The model under review builds one solid part; all positions refer to its coordinate system, in mm. A direction names the side the tool comes from. Give positions to 0.01 mm unless a question says otherwise; leave off trailing zeros. Loops run counter-clockwise (first coordinate to the right, second up) from the corner with the lowest first, then second, coordinate; pieces in that order, holes last. Notation, with made-up numbers: M 3,28.5 L 54,28.5 A25 ccw 54,49.5 Z; hole C -36,77 d6. An arc over 180 degrees is marked long. Put each result on its own line as item: value. Start each with the question number.
```python
from build123d import *

# Parameters (mm, degrees)
SKETCH1_R                     = 3.175
BOSS_EXTRUDE2_DEPTH           = 76.2
SKETCH1_5_R                   = 3.175
BOSS_EXTRUDE3_DEPTH           = 6.35
SKETCH5_R                     = 3.175
BOSS_EXTRUDE4_DEPTH           = 6.35
SKETCH6_W                     = 50.8
SKETCH6_H                     = 50.8
CUT_EXTRUDE1_DEPTH            = 21.59
SKETCH7_W                     = 5.86068256
SKETCH7_H                     = 10.16
BOSS_EXTRUDE5_DEPTH           = 21.59
BOSS_EXTRUDE5_DRAFT           = 5
BOSS_EXTRUDE5_PROFILE_2_DEPTH = 21.59
BOSS_EXTRUDE5_PROFILE_2_DRAFT = 5
BOSS_EXTRUDE5_PROFILE_3_DEPTH = 21.59
BOSS_EXTRUDE5_PROFILE_3_DRAFT = 5
BOSS_EXTRUDE5_PROFILE_4_DEPTH = 21.59
BOSS_EXTRUDE5_PROFILE_4_DRAFT = 5
BOSS_EXTRUDE5_PROFILE_5_DEPTH = 21.59
BOSS_EXTRUDE5_PROFILE_5_DRAFT = 5
SKETCH10_R                    = 36.051864109
CUT_EXTRUDE2_DEPTH            = 21.59


with BuildPart() as part:
    # Sketch1 → Boss-Extrude2 (new body)
    with BuildSketch(Plane(origin=(0, 0, 0), x_dir=(1, 0, 0), z_dir=(0, 1, 0))):
        with BuildLine():
            Line((-4.208751998, -43.475305064), (45.017746951, 2.631829887))
            Line((45.017746951, 2.631829887), (35.550660053, 36.209226482))
            ThreePointArc((35.550660053, 36.209226482), (39.762177432, 42.05307025), (33.11828595, 44.83625091))
            Line((33.11828595, 44.83625091), (15.243844224, 108.232438689))
            Line((15.243844224, 108.232438689), (-2.783728935, 127.479661752))
            Line((-2.783728935, 127.479661752), (3.678966496, 133.532831827))
            Line((3.678966496, 133.532831827), (-3.005742225, 140.669792455))
            Line((-3.005742225, 140.669792455), (-9.468437655, 134.61662238))
            Line((-9.468437655, 134.61662238), (-27.496010814, 153.863845442))
            Line((-27.496010814, 153.863845442), (-74.966911398, 109.401060841))
            Line((-74.966911398, 109.401060841), (-32.227053049, 63.769650553))
            Line((-32.227053049, 63.769650553), (-4.208751998, -43.475305064))
        make_face()
        with Locations(Location((35.334305242, 40.804639607, 0), (0, 0, 90))):
            Circle(SKETCH1_R, mode=Mode.SUBTRACT)
        with BuildLine():
            Line((-27.946524097, 65.532765046), (-68.844709626, 109.197904706))
            Line((-68.844709626, 109.197904706), (-27.496010814, 147.926436632))
            Line((-27.496010814, 147.926436632), (12.111157264, 105.390011693))
            Line((12.111157264, 105.390011693), (34.544848217, 24.491577435))
            ThreePointArc((34.544848217, 24.491577435), (36.285698832, 19.303992732), (36.875100326, 13.863937421))
            ThreePointArc((36.875100326, 13.863937421), (14.585843996, -11.34485616), (-13.162952731, 7.689284266))
            Line((-13.162952731, 7.689284266), (-27.946524097, 65.532765046))
        make_face(mode=Mode.SUBTRACT)
        with Locations(Location((-2.894634056, 134.074815557, 0), (0, 0, 90))):
            Circle(SKETCH1_R, mode=Mode.SUBTRACT)
    extrude(amount=BOSS_EXTRUDE2_DEPTH)

    # Sketch1_5 → Boss-Extrude3 (add)
    with BuildSketch(Plane(origin=(0, 0, 0), x_dir=(1, 0, 0), z_dir=(0, 1, 0))):
        with BuildLine():
            Line((-27.496010814, 147.926436632), (-68.844709626, 109.197904706))
            Line((-68.844709626, 109.197904706), (-27.946524097, 65.532765046))
            Line((-27.946524097, 65.532765046), (-13.162952731, 7.689284266))
            ThreePointArc((-13.162952731, 7.689284266), (3.03743719, 37.821521623), (34.544848217, 24.491577435))
            Line((34.544848217, 24.491577435), (12.111157264, 105.390011693))
            Line((12.111157264, 105.390011693), (-27.496010814, 147.926436632))
        make_face()
        with Locations(Location((-32.808552916, 77.429328599, 0), (0, 0, 270))):
            Circle(SKETCH1_5_R, mode=Mode.SUBTRACT)
        with Locations(Location((-1.199981142, 109.041759799, 0), (0, 0, 270))):
            Circle(SKETCH1_5_R, mode=Mode.SUBTRACT)
    extrude(amount=BOSS_EXTRUDE3_DEPTH)

    # Sketch5 → Boss-Extrude4 (add)
    with BuildSketch(Plane(origin=(0, 76.2, 0), x_dir=(1, 0, 0), z_dir=(0, 1, 0))):
        with BuildLine():
            Line((45.017746951, 2.631829887), (35.550660053, 36.209226482))
            ThreePointArc((35.550660053, 36.209226482), (39.762177432, 42.05307025), (33.11828595, 44.83625091))
            Line((33.11828595, 44.83625091), (15.243844224, 108.232438689))
            Line((15.243844224, 108.232438689), (-2.783728935, 127.479661752))
            Line((-2.783728935, 127.479661752), (3.678966496, 133.532831827))
            Line((3.678966496, 133.532831827), (-3.005742225, 140.669792455))
            Line((-3.005742225, 140.669792455), (-9.468437655, 134.61662238))
            Line((-9.468437655, 134.61662238), (-27.496010814, 153.863845442))
            Line((-27.496010814, 153.863845442), (-74.966911398, 109.401060841))
            Line((-74.966911398, 109.401060841), (-32.227053049, 63.769650553))
            Line((-32.227053049, 63.769650553), (-4.208751998, -43.475305064))
            Line((-4.208751998, -43.475305064), (45.017746951, 2.631829887))
        make_face()
        with Locations(Location((-2.894634056, 134.074815557, 0), (0, 0, 90))):
            Circle(SKETCH5_R, mode=Mode.SUBTRACT)
        with Locations(Location((35.334305242, 40.804639607, 0), (0, 0, 90))):
            Circle(SKETCH5_R, mode=Mode.SUBTRACT)
    extrude(amount=BOSS_EXTRUDE4_DEPTH)

    # Sketch6 → Cut-Extrude1 (cut)
    with BuildSketch(Plane(origin=(14.64974053, 0, -13.721421958), x_dir=(0.683604049055853, 0, 0.729853070223345), z_dir=(-0.729853070223345, 0, 0.683604049055853))):
        with Locations((-99.833701757, 41.275)):
            Rectangle(SKETCH6_W, SKETCH6_H)
    extrude(amount=-CUT_EXTRUDE1_DEPTH, mode=Mode.SUBTRACT)


with BuildPart() as boss_extrude5_tool:
    # Sketch7 → Boss-Extrude5 (with draft: the straight prism first)
    with BuildSketch(Plane(origin=(14.64974053, 0, -13.721421958), x_dir=(0.683604049055853, 0, 0.729853070223345), z_dir=(-0.729853070223345, 0, 0.683604049055853))):
        with Locations((-128.164043037, 77.47)):
            Rectangle(SKETCH7_W, SKETCH7_H)
    extrude(amount=BOSS_EXTRUDE5_DEPTH)
    # Boss-Extrude5: the draft: its side faces are tilted about the plane it starts from
    boss_extrude5_sides = [boss_extrude5_tool.faces().sort_by_distance(p)[0] for p in [
        (-82.845675291, 77.47, -102.021555132),
        (-80.842482126, 72.39, -99.882836552),
        (-78.839288962, 77.47, -97.744117972),
        (-80.842482126, 82.55, -99.882836552),
    ]]
    draft(boss_extrude5_sides, Plane(origin=(14.64974053, 0, -13.721421958), x_dir=(0.683604049055853, 0, 0.729853070223345), z_dir=(-0.729853070223345, 0, 0.683604049055853)), BOSS_EXTRUDE5_DRAFT)


with BuildPart() as part_1:
    add(part.part)

    # Boss-Extrude5: add boss_extrude5_tool
    add(boss_extrude5_tool.part)


with BuildPart() as boss_extrude5_profile_2_tool:
    # Sketch7 → Boss-Extrude5 profile 2 (with draft: the straight prism first)
    with BuildSketch(Plane(origin=(14.64974053, 0, -13.721421958), x_dir=(0.683604049055853, 0, 0.729853070223345), z_dir=(-0.729853070223345, 0, 0.683604049055853))):
        with Locations((-128.164043037, 59.3725)):
            Rectangle(SKETCH7_W, SKETCH7_H)
    extrude(amount=BOSS_EXTRUDE5_PROFILE_2_DEPTH)
    # Boss-Extrude5 profile 2: the draft: its side faces are tilted about the plane it starts from
    boss_extrude5_profile_2_sides = [boss_extrude5_profile_2_tool.faces().sort_by_distance(p)[0] for p in [
        (-80.842482126, 54.2925, -99.882836552),
        (-78.839288962, 59.3725, -97.744117972),
        (-80.842482126, 64.4525, -99.882836552),
        (-82.845675291, 59.3725, -102.021555132),
    ]]
    draft(boss_extrude5_profile_2_sides, Plane(origin=(14.64974053, 0, -13.721421958), x_dir=(0.683604049055853, 0, 0.729853070223345), z_dir=(-0.729853070223345, 0, 0.683604049055853)), BOSS_EXTRUDE5_PROFILE_2_DRAFT)


with BuildPart() as part_2:
    add(part_1.part)

    # Boss-Extrude5 profile 2: add boss_extrude5_profile_2_tool
    add(boss_extrude5_profile_2_tool.part)


with BuildPart() as boss_extrude5_profile_3_tool:
    # Sketch7 → Boss-Extrude5 profile 3 (with draft: the straight prism first)
    with BuildSketch(Plane(origin=(14.64974053, 0, -13.721421958), x_dir=(0.683604049055853, 0, 0.729853070223345), z_dir=(-0.729853070223345, 0, 0.683604049055853))):
        with Locations((-128.164043037, 41.275)):
            Rectangle(SKETCH7_W, SKETCH7_H)
    extrude(amount=BOSS_EXTRUDE5_PROFILE_3_DEPTH)
    # Boss-Extrude5 profile 3: the draft: its side faces are tilted about the plane it starts from
    boss_extrude5_profile_3_sides = [boss_extrude5_profile_3_tool.faces().sort_by_distance(p)[0] for p in [
        (-80.842482126, 36.195, -99.882836552),
        (-78.839288962, 41.275, -97.744117972),
        (-80.842482126, 46.355, -99.882836552),
        (-82.845675291, 41.275, -102.021555132),
    ]]
    draft(boss_extrude5_profile_3_sides, Plane(origin=(14.64974053, 0, -13.721421958), x_dir=(0.683604049055853, 0, 0.729853070223345), z_dir=(-0.729853070223345, 0, 0.683604049055853)), BOSS_EXTRUDE5_PROFILE_3_DRAFT)


with BuildPart() as part_3:
    add(part_2.part)

    # Boss-Extrude5 profile 3: add boss_extrude5_profile_3_tool
    add(boss_extrude5_profile_3_tool.part)


with BuildPart() as boss_extrude5_profile_4_tool:
    # Sketch7 → Boss-Extrude5 profile 4 (with draft: the straight prism first)
    with BuildSketch(Plane(origin=(14.64974053, 0, -13.721421958), x_dir=(0.683604049055853, 0, 0.729853070223345), z_dir=(-0.729853070223345, 0, 0.683604049055853))):
        with Locations((-128.164043037, 23.1775)):
            Rectangle(SKETCH7_W, SKETCH7_H)
    extrude(amount=BOSS_EXTRUDE5_PROFILE_4_DEPTH)
    # Boss-Extrude5 profile 4: the draft: its side faces are tilted about the plane it starts from
    boss_extrude5_profile_4_sides = [boss_extrude5_profile_4_tool.faces().sort_by_distance(p)[0] for p in [
        (-80.842482126, 18.0975, -99.882836552),
        (-78.839288962, 23.1775, -97.744117972),
        (-80.842482126, 28.2575, -99.882836552),
        (-82.845675291, 23.1775, -102.021555132),
    ]]
    draft(boss_extrude5_profile_4_sides, Plane(origin=(14.64974053, 0, -13.721421958), x_dir=(0.683604049055853, 0, 0.729853070223345), z_dir=(-0.729853070223345, 0, 0.683604049055853)), BOSS_EXTRUDE5_PROFILE_4_DRAFT)


with BuildPart() as part_4:
    add(part_3.part)

    # Boss-Extrude5 profile 4: add boss_extrude5_profile_4_tool
    add(boss_extrude5_profile_4_tool.part)


with BuildPart() as boss_extrude5_profile_5_tool:
    # Sketch7 → Boss-Extrude5 profile 5 (with draft: the straight prism first)
    with BuildSketch(Plane(origin=(14.64974053, 0, -13.721421958), x_dir=(0.683604049055853, 0, 0.729853070223345), z_dir=(-0.729853070223345, 0, 0.683604049055853))):
        with Locations((-128.164043037, 5.08)):
            Rectangle(SKETCH7_W, SKETCH7_H)
    extrude(amount=BOSS_EXTRUDE5_PROFILE_5_DEPTH)
    # Boss-Extrude5 profile 5: the draft: its side faces are tilted about the plane it starts from
    boss_extrude5_profile_5_sides = [boss_extrude5_profile_5_tool.faces().sort_by_distance(p)[0] for p in [
        (-80.842482126, 0, -99.882836552),
        (-78.839288962, 5.08, -97.744117972),
        (-80.842482126, 10.16, -99.882836552),
        (-82.845675291, 5.08, -102.021555132),
    ]]
    draft(boss_extrude5_profile_5_sides, Plane(origin=(14.64974053, 0, -13.721421958), x_dir=(0.683604049055853, 0, 0.729853070223345), z_dir=(-0.729853070223345, 0, 0.683604049055853)), BOSS_EXTRUDE5_PROFILE_5_DRAFT)


with BuildPart() as part_5:
    add(part_4.part)

    # Boss-Extrude5 profile 5: add boss_extrude5_profile_5_tool
    add(boss_extrude5_profile_5_tool.part)

    # Sketch10 → Cut-Extrude2 (cut)
    with BuildSketch(Plane(origin=(-89.616651928, 0, -95.679638883), x_dir=(-0.7298530702233451, 0, 0.683604049055853), z_dir=(-0.683604049055853, 0, -0.7298530702233451))):
        with Locations((29.820674878, 41.547690044)):
            Circle(SKETCH10_R)
    extrude(amount=-CUT_EXTRUDE2_DEPTH, mode=Mode.SUBTRACT)


solid = part_5.part
```
Item 1: Tool access review of faces 4 (the flat face through (-78.057, 36.802, -102.548)), 5 (the flat face through (-76.441, 41.204, -100.822)), 6 (the flat face through (-6.19, 40.7, -137.69)): name each direction out of +Z, -Z, +X, -X, +Y, -Y from which nothing blocks a thin tool from reaching the whole face with its end or side.
Item 2: Consider section C-C, the plane y = 49.5. Give the number of separate pieces and of enclosed holes in the cut face, plus the area to 3 significant figures.
Item 3: Consider section A-A, the plane z = -118. Write out the cut boundary in (x, y), plus the area to 3 significant figures.
Item 4: Consider section D-D, the plane x = -45.5. Write out the cut boundary in (y, z) (3 decimals).
Item 5: Clearance check with flat-ended pins moving along their axes: pin 1 Ø4 at (x, y) = (-74, 47) entering from +Z; pin 2 Ø4 at (x, y) = (19.5, 47) entering from +Z; pin 3 Ø10 at (x, z) = (1.5, -23.5) entering from -Y. State where each tip first meets the part, or that it passes through.
Item 6: Consider section B-B, the plane x = -21. Write out the cut boundary in (y, z), plus the area to 3 significant figures.
Item 7: Draft analysis for pull direction X (two halves, no side actions). For faces 1 (the flat face through (-31.638, 38.525, -69.474)), 2 (the flat face through (-78.75, 63.762, -101.899)), 3 (the flat face through (0.4, 40.7, -130.46)), state which applies: +X half, -X half, draft (parallel to the pull), parting line (faces both ways), or undercut.
Item 8: To check wall thickness, follow L1, parallel to Y at x = -36, z = -92; L2, parallel to Z at x = -4, y = 76; L3, parallel to Z at x = -41, y = 6.5. State the ranges of each line that lie inside material, in increasing order. Write a range as [from, to].
Report:
1. face 4: +Z, -X
1. face 5: +Z, +Y, -Y
1. face 6: -Z, +Y, -Y
2. separate pieces: 1
2. enclosed holes: 2
2. area: 2,330 mm²
3. outline: M -65.79,0 L 6.1,0 L 6.1,82.55 L -65.79,82.55 Z; hole M -59.45,6.35 L 0.37,6.35 L 0.37,76.2 L -59.45,76.2 Z
3. area: 1,760 mm²
4. outline: M 0,-137.001 L 82.55,-137.001 L 82.55,-77.941 L 66.675,-77.941 L 66.675,-84.274 L 76.2,-84.274 L 76.2,-131.063 L 6.35,-131.063 L 6.35,-84.274 L 15.875,-84.274 L 15.875,-77.941 L 0,-77.941 Z
5. pin 1: z = -101.46
5. pin 2: z = 23.14
5. pin 3: y = 76.2
6. outline: M 0,-146.93 L 82.55,-146.93 L 82.55,-20.8 L 0,-20.8 Z; hole M 6.35,-140.95 L 76.2,-140.95 L 76.2,-38.35 L 6.35,-38.35 Z
6. area: 3,250 mm²
7. face 1: undercut
7. face 2: -X half
7. face 3: +X half
8. L1: [0, 6.35], [76.2, 82.55]
8. L2: [-139.74, -137.05], [-131.1, -122.69], [6.28, 43.28]
8. L3: [-141.22, -135.28], [-79.47, -73.14]
